Work out the finished part from the listing and answer in its coordinate system (mm). A direction names the side the tool comes from. Round coordinates to 2 decimals unless told otherwise and drop trailing zeros. Loops run counter-clockwise (first coordinate to the right, second up) from the corner with the lowest first, then second, coordinate; pieces in that order, holes last.
Autodesk Inventor part; units mm, degrees
ref_plane "Work Plane1" through (1.525, 0, 0) normal (0, 0, 1) x (1, 0, 0)
ref_plane "YZ Plane" through (0, 0, 0) normal (1, 0, 0) x (0, 1, 0)
ref_plane "XZ Plane" through (0, 0, 0) normal (0, 1, 0) x (-1, 0, 0)
sketch "Skizze1" plane through (0, 0, 0) normal (0, 0, 1) x (1, 0, 0)
  line L0 (0, 7.7) -> (0, 5)
  line L1 (3, 5) -> (140, 5)
  line L2 (140, 5) -> (140, 0)
  line L3 (140, 0) -> (-0.6001, 0)
  line L4 (-28.7201, 0) -> (168.12, 0)
  line L5 (-0.6001, 0) -> (-0.6001, 7.7)
  line L6 (-0.6001, 7.7) -> (0, 7.7)
  line L7 (3, 5) -> (2.3864, 5)
  line L8 (2.3864, 5) -> (0, 5)
  line L9 (0, -1.54) -> (0, 9.24)
  dimension "d0" = 140
  dimension "d1" = 137
  dimension "d2" = 10
  dimension "d9" = 0.6001
  dimension "d10" = 15.4
  dimension "d13" = 0.6136
  dimension "d14" = 10
revolve "Körper" add sketch "Skizze1" angle 360 about axis through (140, 0, 0) along (-1, 0, 0)
sketch "Skizze2" plane through (-0.6001, 0, 0) normal (-1, 0, 0) x (0, 0, 1)
  line L0 (0, 9.815) -> (8.5, 4.9075)
  line L1 (8.5, 4.9075) -> (8.5, -4.9075)
  line L2 (8.5, -4.9075) -> (0, -9.815)
  line L3 (0, -9.815) -> (-8.5, -4.9075)
  line L4 (-8.5, -4.9075) -> (-8.5, 4.9075)
  line L5 (-8.5, 4.9075) -> (0, 9.815)
  point P0 (0, 0)
  point P1 (0, 0)
  dimension "d11" = 17
extrude "Kopf" add sketch "Skizze2" along normal blind 5.8
sketch "Skizze4" plane through (0, 0, 0) normal (0, 0, 1) x (1, 0, 0)
  line L0 (-6.4001, 8.5) -> (-6.4001, 9.815)
  line L1 (-6.4001, 9.815) -> (-5.6409, 9.815)
  line L2 (-5.6409, 9.815) -> (-6.4001, 8.5)
  line L3 (-7.5601, 0) -> (0.5599, 0)
  line L4 (-0.6001, 9.815) -> (-6.4001, 9.815)
  line L5 (-6.4001, 4.9075) -> (-6.4001, 9.815)
  dimension "d5" = 30
  dimension "d19" = 17
revolve "Fase1" cut sketch "Skizze4" angle 360 about axis through (-10, 0, 0) along (1, 0, 0)
thread "Gewinde"
chamfer "Fase2" distance 0.6134 distance2 0.6136 1 edges at (140, -5, 0) measured on face at (140, 2.3641, -0.6817)
ref_plane "Work Plane1" through (1.525, 0, 0) normal (0, 0, 1) x (1, 0, 0)
equation "\"d0\" = NLG"
equation "\"d1\" = GEL"
equation "\"d2\" = GD"
equation "\"d10\" = SD2"
equation "\"d14\" = BDM"
equation "\"d11\" = SW"
equation "\"d3\" = KOH - SD"
equation "\"d5\" = ANG1"
equation "\"d19\" = SW0"
equation "\"d15\" = GEL"
equation "\"d6\" = -0.5 * SPD + 0.5 * GD"
equation "\"NLG\" = 140"
equation "\"GD\" = NND"
equation "\"BDM\" = NND"
equation "\"KOH\" = 6.4"
equation "\"GEL\" = 137"
equation "\"SW\" = 17"
equation "\"SW0\" = 17"
equation "\"SPD\" = NND - 1.2269 * PTC"
equation "\"SD2\" = 15.4"
equation "\"SD\" = 0.6"
equation "\"ANG1\" = 30deg"
equation "\"GAL\" = 0.61345 * PTC"
equation "\"GUL\" = 0.61345 * PTC"
equation "\"RR\" = 0"
equation "\"GD1\" = THREADDIA - 1.2269 * PTC"
equation "\"TOA\" = 30deg"
equation "\"FAWI\" = 45deg"
equation "\"PTC\" = 1"
equation "\"E0\" = 1.155 * SW"
properties part number "DIN 961 - M10 x 140" material "Stahl, weich"
Item 1: Straight lines are drawn through the part: line 1 (X direction, y = 8, z = 1); line 2 (Z direction, x = 45.5, y = 0); line 3 (X direction, y = 1.25, z = -7). For each, find the intervals that lie inside material, in ascending order.
Item 2: Section A-A, the plane x = 59.5 is taken. Give the vertices of the cut face in (y, z), plus the area to 3 significant figures.
Item 3: For faces 1 (the face through (-3, 0, -8.5)), 2 (the face through (-0.296, -1.669, -7.517)), determine the directions among +Z, -Z, +X, -X, +Y, -Y from which every point of the face is accessible in a straight line to the end or side of a thin tool.
Item 4: Each of these flat-tipped pins is pushed along its axis until it touches: P1, Ø3, axis at x = 68.5, y = 6, coming from the -Z side; P2, Ø10, axis at y = 7.5, z = 4, coming from the +X side; P3, Ø1, axis at y = 1.5, z = -5, coming from the +X side; P4, Ø1, axis at x = 119, z = 0, coming from the +Y side. Where does it stop, or does it pass through?
Answer below:
1. line 1: x = -6.4 to -0.6
1. line 2: z = -5 to 5
1. line 3: x = -6.4 to 0
2. outline: circle Ø10 at (0, 0)
2. area: 78.5 mm2
3. face 1: -Z, +X, -X, +Y, -Y
3. face 2: +X
4. P1: stops at z = -2.18
4. P2: stops at x = 140
4. P3: stops at x = 139.67
4. P4: stops at y = 5
